Can you work these out from the model? Positions are in its coordinate system, mm. A direction names the side the tool comes from. Give positions to 0.01 mm unless a question says otherwise; leave off trailing zeros. Order: outer loops, then holes, each group sorted by start corner. A loop starts at its lowest first (then second) coordinate and runs counter-clockwise, first axis right, second up. Notation, with made-up numbers: (37.5, 28) - (46.5, 28) arc R19 cw to (46.5, 43) - close; hole circle Ø5 at (-37.5, 44.5). An arc over 180 degrees is marked (long way). Answer as CSV lines item,"result".
```python
from build123d import *

# Parameters (mm, degrees)
FILLET1_R = 0.2


with BuildPart() as part:
    # Sketch1 → Revolve1 (revolve)
    with BuildSketch(Plane.XY):
        Polygon((3, 1), (3, 7.5), (4, 7.5), (4, 6.7), (4.5, 6.7), (4.5, 6.5), (4, 6.5), (4, 3), (4.1, 3), (4.1, 1.5), (5, 1.5), (5, 1), align=None)
    revolve(axis=Axis((0, 0, 0), (1, 0, 0)))

    # Fillet1
    fillet1_edges = [part.edges().sort_by_distance(p)[0] for p in [
        (4, -7.5, 0),
    ]]
    fillet(fillet1_edges, radius=FILLET1_R)


solid = part.part
```
1) I'm going to push flat-ended pins straight in: P1, Ø1, axis at x = 4, z = -2, coming from the +Y side; P2, Ø1.8, axis at y = 0, z = 0, coming from the +X side. Where does each tip first touch, or does it pass through?
Answer block:
P1,"y = 7.34"
P2,"through"
2) I need wall thicknesses on line 1 along Z through (x, y) = (4.25, 0); line 2 along Y through (x, z) = (4.4, -0.5); line 3 along Z through (x, y) = (3.35, 0). Which ranges of each line are inside material? Lowest first, please. Write a range as [from, to].
Answer block:
line 1,"[-6.7, -6.5], [-1.5, -1], [1, 1.5], [6.5, 6.7]"
line 2,"[-6.68, -6.48], [-1.41, -0.87], [0.87, 1.41], [6.48, 6.68]"
line 3,"[-7.5, -1], [1, 7.5]"
3) Which directions (+Z, -Z, +X, -X, +Y, -Y) give clear straight access to the entire face, cutting with the end or side of a thin tool? Please do faces 1 (the cylindrical face through (4.246, -5.158, -3.955)), 2 (the cylindrical face through (4, 0, -1)).
Answer block:
face 1,"+X"
face 2,"+X, -X"
4) I want a section at A-A on z = 0. Write out the boundary of the cut face in (x, y).
Answer block:
outline,"(3, -7.5) - (3.8, -7.5) arc R0.2 ccw to (4, -7.3) - (4, -6.7) - (4.5, -6.7) - (4.5, -6.5) - (4, -6.5) - (4, -3) - (4.1, -3) - (4.1, -1.5) - (5, -1.5) - (5, -1) - (3, -1) - close; (3, 1) - (5, 1) - (5, 1.5) - (4.1, 1.5) - (4.1, 3) - (4, 3) - (4, 6.5) - (4.5, 6.5) - (4.5, 6.7) - (4, 6.7) - (4, 7.3) arc R0.2 ccw to (3.8, 7.5) - (3, 7.5) - close"
5) I want a section at B-B on x = 3.2. Write out the boundary of the cut face in (y, z), plus the area to 3 significant figures.
Answer block:
outline,"circle Ø15 at (0, 0); hole circle Ø2 at (0, 0)"
area,"174 mm2"
6) If we mould it in two halves opening along Y, with no side actions, what happens to faces 3 (the cylindrical face through (3.406, -7.493, 0.33)), 4 (the flat face through (3, 0, -2)), 5 (the flat face through (4.1, 1.3, -1.3)), 6 (the flat face through (4, 3, -1))? For each: +Y half, -Y half, draft (parallel to the pull), parting line (faces both ways), or undercut.
Answer block:
face 3,"parting line"
face 4,"draft"
face 5,"undercut"
face 6,"undercut"
